Input: dimensioned drawing with shaded views. Units: mm. Origin: part minimum x, y, z. Coordinates: 2 decimals unless noted, no trailing zeros. Order: outer loops, then holes, each group sorted by start corner. A loop starts at its lowest first (then second) coordinate and runs counter-clockwise, first axis right, second up. Notation, with made-up numbers: (34.25, -1.75) -> (88.25, -1.75) arc R18 cw to (88.25, 10.25) -> close; hole circle Ø9 at (-30.75, 4). An arc over 180 degrees is marked (long way). Answer in a Markdown table with one row per item. Add a question column.
1) Section query B-B on y = 20. Return the cut outline in (x, z), then the cut area to 3 significant figures.
2) Pull-direction query (Y, two-part tool) for the marked faces 1, 2 and 3; classes: +Y half, -Y half, draft (parallel to the pull), parting line (faces both ways), or undercut.
3) Section query C-C on z = 4. Count the separate pieces of the cut face and the enclosed holes in it, then the cut area to 3 significant figures.
4) Contact query for a flat-ended pin moving along its axis: P1, Ø3.5, axis at x = 8.5, z = 4, coming from the -Y side. Output: stop coordinate, or through.
5) Section query D-D on y = 57. Return the cut outline in (x, z).
6) Section query A-A on x = 83.5. Return the cut outline in (y, z).
7) Ray query, line 1 (Y direction, x = 83.5, z = 5.25); line 2 (X direction, y = 21, z = 4.75); line 3 (X direction, y = 60, z = 1). Return the intervals inside material, ascending. Write a range as from..to.
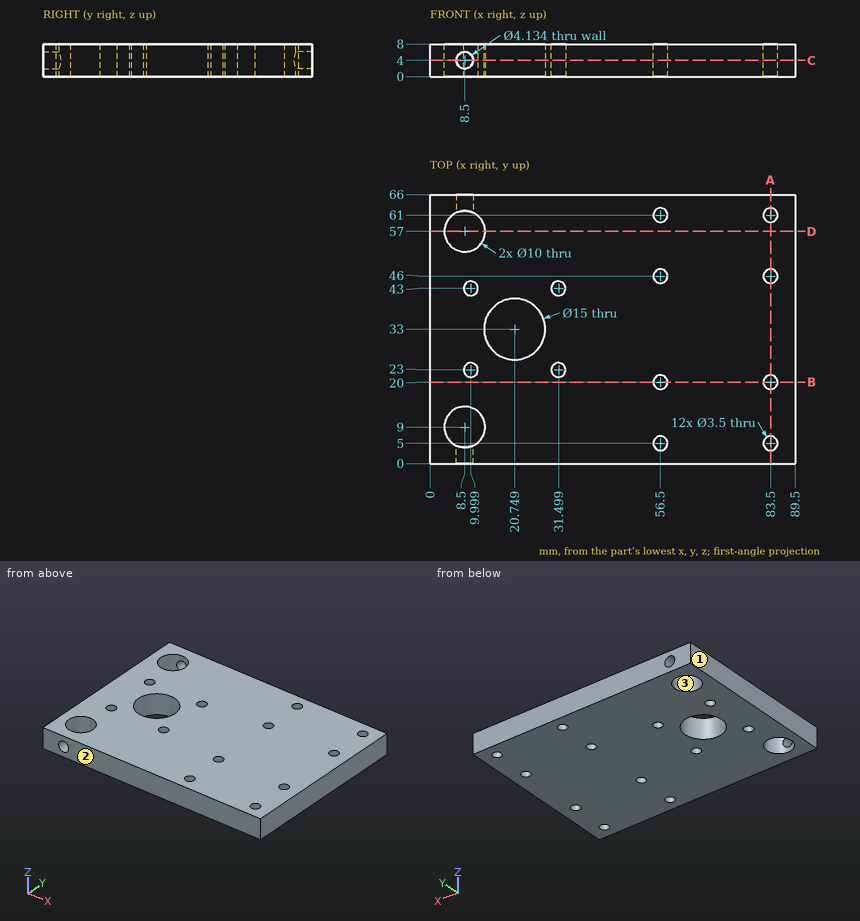
Result:
| question | item | result |
|---|---|---|
| 1 | outline | (0, 0) -> (54.75, 0) -> (54.75, 8) -> (0, 8) -> close; (58.25, 0) -> (81.75, 0) -> (81.75, 8) -> (58.25, 8) -> close; (85.25, 0) -> (89.5, 0) -> (89.5, 8) -> (85.25, 8) -> close |
| 1 | area | 660 mm2 |
| 2 | face 1 | draft |
| 2 | face 2 | -Y half |
| 2 | face 3 | undercut |
| 3 | separate pieces | 1 |
| 3 | enclosed holes | 13 |
| 3 | area | 5,420 mm2 |
| 4 | P1 | y = 13.68 |
| 5 | outline | (0, 0) -> (3.5, 0) -> (3.5, 8) -> (0, 8) -> close; (13.5, 0) -> (89.5, 0) -> (89.5, 8) -> (13.5, 8) -> close |
| 6 | outline | (0, 0) -> (3.25, 0) -> (3.25, 8) -> (0, 8) -> close; (6.75, 0) -> (18.25, 0) -> (18.25, 8) -> (6.75, 8) -> close; (21.75, 0) -> (44.25, 0) -> (44.25, 8) -> (21.75, 8) -> close; (47.75, 0) -> (59.25, 0) -> (59.25, 8) -> (47.75, 8) -> close; (62.75, 0) -> (66, 0) -> (66, 8) -> (62.75, 8) -> close |
| 7 | line 1 | 0..3.25, 6.75..18.25, 21.75..44.25, 47.75..59.25, 62.75..66 |
| 7 | line 2 | 0..55.06, 57.94..82.06, 84.94..89.5 |
| 7 | line 3 | 0..4.5, 12.5..55.06, 57.94..82.06, 84.94..89.5 |
